Can you work these out from the model? Positions are in its coordinate system, mm. A direction names the side the tool comes from. Give positions to 0.01 mm unless a question says otherwise; leave off trailing zeros. Loops run counter-clockwise (first coordinate to the right, second up) from the corner with the lowest first, then second, coordinate; pieces in that order, holes last. Notation, with made-up numbers: (35, 24) -> (89, 24) arc R28 ccw to (89, 42) -> close; hole circle Ø1 at (74, 44). An arc over 180 degrees is marked (long way). Return JSON: item names as keys, results as strings. Group by question number.
Q1. Which directions (+Z, -Z, +X, -X, +Y, -Y) give clear straight access to the entire face, cutting with the end or side of a thin tool? Please do faces 1 (the flat face through (49, 1, 0)), 2 (the flat face through (75, 1, -12.1)).
Q2. Suppose I cut it at B-B, the plane x = 27.5. Please give me the cut outline in (y, z), and give its area (3 significant figures).
Q3. Suppose I cut it at D-D, the plane z = -40.5. Please give me the cut outline in (x, y), and give its area (3 significant figures).
Q4. Suppose I cut it at A-A, the plane z = -25. Please give me the cut outline in (x, y).
Q5. I need wall thicknesses on line 1 along Z through (x, y) = (80, 0.4); line 2 along X through (y, z) = (2.4, -25); line 3 along Z through (x, y) = (36.5, 1). Which ranges of each line are inside material? Lowest first, please. Write a range as [from, to].
Q6. Suppose I cut it at C-C, the plane y = 0.8. Please give me the cut outline in (x, z).
```python
from build123d import *

# Parameters (mm, degrees)
SKETCH_1_W      = 100
SKETCH_1_H      = 50
SKETCH_1_R      = 11
SKETCH_1_R_2    = 1.6
EXTRUDE_1_DEPTH = 3
CHAMFER_1_SIZE  = 6


with BuildPart() as part:
    # 草图1 → 凸台-拉伸1 (new body)
    with BuildSketch(Plane(origin=(0, 0, 0), x_dir=(1, 0, 0), z_dir=(0, 1, 0))):
        with Locations((50, 25)):
            Rectangle(SKETCH_1_W, SKETCH_1_H)
        with Locations((21, 25)):
            Circle(SKETCH_1_R, mode=Mode.SUBTRACT)
        with Locations((5.5, 40.5)):
            Circle(SKETCH_1_R_2, mode=Mode.SUBTRACT)
        with Locations((36.5, 40.5)):
            Circle(SKETCH_1_R_2, mode=Mode.SUBTRACT)
        with Locations((36.5, 9.5)):
            Circle(SKETCH_1_R_2, mode=Mode.SUBTRACT)
        with Locations((5.5, 9.5)):
            Circle(SKETCH_1_R_2, mode=Mode.SUBTRACT)
        with BuildLine():
            Line((60, 42.1), (90, 42.1))
            ThreePointArc((90, 42.1), (92.1, 40), (90, 37.9))
            Line((90, 37.9), (60, 37.9))
            ThreePointArc((60, 37.9), (57.9, 40), (60, 42.1))
        make_face(mode=Mode.SUBTRACT)
        with BuildLine():
            Line((60, 7.9), (90, 7.9))
            ThreePointArc((90, 7.9), (92.1, 10), (90, 12.1))
            Line((90, 12.1), (60, 12.1))
            ThreePointArc((60, 12.1), (57.9, 10), (60, 7.9))
        make_face(mode=Mode.SUBTRACT)
    extrude(amount=EXTRUDE_1_DEPTH)

    # 倒角1
    chamfer_1_edges = [part.edges().sort_by_distance(p)[0] for p in [
        (0, 1.5, -50),
        (100, 1.5, -50),
        (100, 1.5, 0),
        (0, 1.5, 0),
    ]]
    chamfer(chamfer_1_edges, length=CHAMFER_1_SIZE)


solid = part.part
```
Ans:
{
 "1": {"face 1": "+Z, +X, -X, +Y, -Y", "face 2": "+Y, -Y"},
 "2": {"outline": "(0, -50) -> (3, -50) -> (3, -33.87) -> (0, -33.87) -> close; (0, -16.13) -> (3, -16.13) -> (3, 0) -> (0, 0) -> close", "area": "96.8 mm^2"},
 "3": {"outline": "(0, 0) -> (3.9, 0) -> (3.9, 3) -> (0, 3) -> close; (7.1, 0) -> (34.9, 0) -> (34.9, 3) -> (7.1, 3) -> close; (38.1, 0) -> (57.96, 0) -> (57.96, 3) -> (38.1, 3) -> close; (92.04, 0) -> (100, 0) -> (100, 3) -> (92.04, 3) -> close", "area": "179 mm^2"},
 "4": {"outline": "(0, 0) -> (10, 0) -> (10, 3) -> (0, 3) -> close; (32, 0) -> (100, 0) -> (100, 3) -> (32, 3) -> close"},
 "5": {"line 1": "z = [-50, -42.1], [-37.9, -12.1], [-7.9, 0]", "line 2": "x = [0, 10], [32, 100]", "line 3": "z = [-50, -42.1], [-38.9, -11.1], [-7.9, 0]"},
 "6": {"outline": "(0, -44) -> (6, -50) -> (94, -50) -> (100, -44) -> (100, -6) -> (94, 0) -> (6, 0) -> (0, -6) -> close; hole circle Ø3.2 at (5.5, -40.5); hole circle Ø3.2 at (5.5, -9.5); hole circle Ø22 at (21, -25); hole circle Ø3.2 at (36.5, -40.5); hole circle Ø3.2 at (36.5, -9.5); hole (60, -42.1) -> (90, -42.1) arc R2.1 ccw to (90, -37.9) -> (60, -37.9) arc R2.1 ccw to start; hole (60, -12.1) -> (90, -12.1) arc R2.1 ccw to (90, -7.9) -> (60, -7.9) arc R2.1 ccw to start"}
}
